For this review, take the finished solid that the model builds, in its own axes (mm). Face numbers are marked on the shaded views. Round coordinates to 2 decimals unless told otherwise and drop trailing zeros. Order: outer loops, then holes, each group sorted by start corner. A loop starts at its lowest first (then second) coordinate and runs counter-clockwise, first axis right, second up. Notation, with made-up numbers: (-22.5, 54.25) -> (17.5, 54.25) arc R27 cw to (17.5, 73.25) -> close; hole circle Ø3 at (55, 78). An arc over 180 degrees is marked (long way). Answer in a Markdown table with one row per item.
```python
from build123d import *

# Parameters (mm, degrees)
SKETCH1_W           = 99
SKETCH1_H           = 51
BOSS_EXTRUDE2_DEPTH = 31
CUT_EXTRUDE1_DEPTH  = 96
SKETCH4_W           = 3
SKETCH4_H           = 31
CUT_EXTRUDE2_DEPTH  = 3
SKETCH6_W           = 2
SKETCH6_H           = 2
BOSS_EXTRUDE3_DEPTH = 96
SKETCH7_W           = 1
SKETCH7_H           = 1
CUT_EXTRUDE3_DEPTH  = 45
FILLET1_R           = 3
SKETCH9_R           = 1
SKETCH9_R_2         = 0.5
CUT_EXTRUDE4_DEPTH  = 10


with BuildPart() as part:
    # Sketch1 → Boss-Extrude2 (new body)
    with BuildSketch(Plane.XY):
        Rectangle(SKETCH1_W, SKETCH1_H)
    extrude(amount=BOSS_EXTRUDE2_DEPTH)

    # Sketch3 → Cut-Extrude1 (cut)
    with BuildSketch(Plane.ZY.offset(49.5)):
        Polygon((3, 0.616456183), (3, -22.5), (28, -22.5), (28, 22.5), (3, 22.5), align=None)
    extrude(amount=-CUT_EXTRUDE1_DEPTH, mode=Mode.SUBTRACT)

    # Sketch4 → Cut-Extrude2 (cut)
    with BuildSketch(Plane.XZ.offset(25.5)):
        with Locations((-48, 15.5)):
            Rectangle(SKETCH4_W, SKETCH4_H)
    extrude(amount=-CUT_EXTRUDE2_DEPTH, mode=Mode.SUBTRACT)

    # Sketch6 → Boss-Extrude3 (add)
    with BuildSketch(Plane.ZY.offset(46.5)):
        with Locations((13.2, -21.5)):
            Rectangle(SKETCH6_W, SKETCH6_H)
        with Locations((17.8, -21.5)):
            Rectangle(SKETCH6_W, SKETCH6_H)
        with Locations((13.2, 21.5)):
            Rectangle(SKETCH6_W, SKETCH6_H)
        with Locations((17.8, 21.5)):
            Rectangle(SKETCH6_W, SKETCH6_H)
    extrude(amount=-BOSS_EXTRUDE3_DEPTH)

    # Sketch7 → Cut-Extrude3 (cut)
    with BuildSketch(Plane.XZ.offset(22.5)):
        with Locations((-48.055142405, 28.5)):
            Rectangle(SKETCH7_W, SKETCH7_H)
        with Locations((-48.055142405, 2.5)):
            Rectangle(SKETCH7_W, SKETCH7_H)
    extrude(amount=-CUT_EXTRUDE3_DEPTH, mode=Mode.SUBTRACT)

    # Fillet1
    fillet1_edges = [part.edges().sort_by_distance(p)[0] for p in [
        (0, 25.5, 31),
        (1.5, -25.5, 31),
        (1.5, -25.5, 0),
        (0, 25.5, 0),
    ]]
    fillet(fillet1_edges, radius=FILLET1_R)

    # Sketch9 → Cut-Extrude4 (cut)
    # profile 1 of 8: a face of its own
    with BuildSketch(Plane(origin=(0, 0, 28), x_dir=(-1, 0, 0), z_dir=(0, 0, -1))):
        with BuildLine():
            ThreePointArc((-43.107346254, 2.807819217), (-44.043005412, 0.051456221), (-43.107346254, -2.704906774))
            ThreePointArc((-43.107346254, -2.704906774), (-42.125865916, -2.834121112), (-41.996651578, -1.852640773))
            ThreePointArc((-41.996651578, -1.852640773), (-42.643005412, 0.051456221), (-41.996651578, 1.955553216))
            ThreePointArc((-41.996651578, 1.955553216), (-42.125865916, 2.937033554), (-43.107346254, 2.807819217))
        make_face()
    # profile 2 of 8: a face of its own
    with BuildSketch(Plane(origin=(0, 0, 28), x_dir=(-1, 0, 0), z_dir=(0, 0, -1))):
        with BuildLine():
            ThreePointArc((-37.730978714, 6.710201232), (-42.153265918, 6.420349215), (-45.485251514, 3.498276272))
            ThreePointArc((-45.485251514, 3.498276272), (-45.229033732, 2.542058489), (-44.272815949, 2.798276272))
            ThreePointArc((-44.272815949, 2.798276272), (-41.617509112, 5.12691787), (-38.093325377, 5.357905075))
            ThreePointArc((-38.093325377, 5.357905075), (-37.236003967, 5.852879822), (-37.730978714, 6.710201232))
        make_face()
    # profile 3 of 8: a face of its own
    with BuildSketch(Plane(origin=(0, 0, 28), x_dir=(-1, 0, 0), z_dir=(0, 0, -1))):
        with BuildLine():
            ThreePointArc((-35.59397575, 2.315366896), (-35.850193532, 1.359149114), (-36.806411315, 1.615366896))
            ThreePointArc((-36.806411315, 1.615366896), (-38.318218652, 2.941186348), (-40.324723797, 3.072699643))
            ThreePointArc((-40.324723797, 3.072699643), (-41.182045207, 3.56767439), (-40.68707046, 4.4249958))
            ThreePointArc((-40.68707046, 4.4249958), (-37.782461847, 4.234617693), (-35.59397575, 2.315366896))
        make_face()
    # profile 4 of 8: a face of its own
    with BuildSketch(Plane(origin=(0, 0, 28), x_dir=(-1, 0, 0), z_dir=(0, 0, -1))):
        with BuildLine():
            ThreePointArc((-34.046091661, -4.145125978), (-32.621543961, 0.051456221), (-34.046091661, 4.24803842))
            ThreePointArc((-34.046091661, 4.24803842), (-35.027572, 4.377252758), (-35.156786338, 3.39577242))
            ThreePointArc((-35.156786338, 3.39577242), (-34.021543961, 0.051456221), (-35.156786338, -3.292859977))
            ThreePointArc((-35.156786338, -3.292859977), (-35.027572, -4.274340315), (-34.046091661, -4.145125978))
        make_face()
    # profile 5 of 8: a face of its own
    with BuildSketch(Plane(origin=(0, 0, 28), x_dir=(-1, 0, 0), z_dir=(0, 0, -1))):
        with BuildLine():
            ThreePointArc((-40.203971578, -4.423668127), (-37.337352845, -3.918205901), (-35.370817206, -1.772108839))
            ThreePointArc((-35.370817206, -1.772108839), (-35.729612558, -0.849468121), (-36.652253276, -1.208263474))
            ThreePointArc((-36.652253276, -1.208263474), (-38.010737122, -2.690788443), (-39.990998837, -3.039962012))
            ThreePointArc((-39.990998837, -3.039962012), (-40.789338265, -3.625328699), (-40.203971578, -4.423668127))
        make_face()
    # profile 6 of 8: a face of its own
    with BuildSketch(Plane(origin=(0, 0, 28), x_dir=(-1, 0, 0), z_dir=(0, 0, -1))):
        with BuildLine():
            ThreePointArc((-46.089765479, -2.021501337), (-45.632657673, -1.143405411), (-44.754561748, -1.600513217))
            ThreePointArc((-44.754561748, -1.600513217), (-42.666206574, -4.448670298), (-39.275554847, -5.436955151))
            ThreePointArc((-39.275554847, -5.436955151), (-38.54568752, -6.105755335), (-39.214487704, -6.835622662))
            ThreePointArc((-39.214487704, -6.835622662), (-43.469213585, -5.59548316), (-46.089765479, -2.021501337))
        make_face()
    # profile 7 of 8: a face of its own
    with BuildSketch(Plane(origin=(0, 0, 28), x_dir=(-1, 0, 0), z_dir=(0, 0, -1))):
        with Locations((-39.515184062, 0.051456221)):
            Circle(SKETCH9_R)
        with Locations((-39.515184062, 0.051456221)):
            Circle(SKETCH9_R_2, mode=Mode.SUBTRACT)
    # profile 8 of 8: a face of its own
    with BuildSketch(Plane(origin=(0, 0, 28), x_dir=(-1, 0, 0), z_dir=(0, 0, -1))):
        with Locations((-39.515184062, 0.051456221)):
            Circle(SKETCH9_R_2)
    extrude(amount=-CUT_EXTRUDE4_DEPTH, mode=Mode.SUBTRACT)


solid = part.part
```
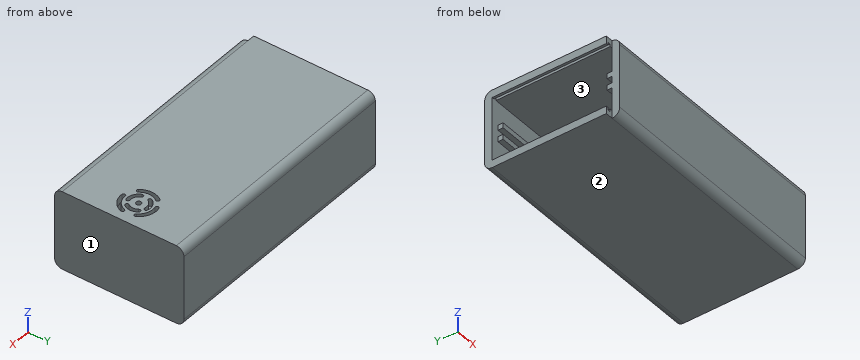
Q1. To check wall thickness, follow probe 1 along Y at (x, z) = (-32.5, 22); probe 2 along Z at (x, y) = (-42.5, -22); probe 3 along Z at (x, y) = (28, 8). State the ranges of each line that lie inside material, in increasing order.
Answer key:
| item | result |
|---|---|
| probe 1 | y = -25.5 to -22.5, 22.5 to 25.5 |
| probe 2 | z = 0 to 3, 12.2 to 14.2, 16.8 to 18.8, 28 to 31 |
| probe 3 | z = 0 to 3, 28 to 31 |
Q2. Take a section at A-A, the plane x = -12.5. Write out the cut boundary in (y, z).
Answer key:
| item | result |
|---|---|
| outline | (-25.5, 3) arc R3 ccw to (-22.5, 0) -> (22.5, 0) arc R3 ccw to (25.5, 3) -> (25.5, 28) arc R3 ccw to (22.5, 31) -> (-22.5, 31) arc R3 ccw to (-25.5, 28) -> close; hole (-22.5, 3) -> (22.5, 3) -> (22.5, 12.2) -> (20.5, 12.2) -> (20.5, 14.2) -> (22.5, 14.2) -> (22.5, 16.8) -> (20.5, 16.8) -> (20.5, 18.8) -> (22.5, 18.8) -> (22.5, 28) -> (-22.5, 28) -> (-22.5, 18.8) -> (-20.5, 18.8) -> (-20.5, 16.8) -> (-22.5, 16.8) -> (-22.5, 14.2) -> (-20.5, 14.2) -> (-20.5, 12.2) -> (-22.5, 12.2) -> close |
Q3. Clearance check with flat-ended pins moving along their axes: pin 1 Ø0.9 at (x, z) = (-47.5, 1) entering from -Y; pin 2 Ø4 at (y, z) = (18.5, 21) entering from -X; pin 3 Ø2 at (y, z) = (21, 17.5) entering from -X. State where each tip first meets the part, or that it passes through.
Answer key:
| item | result |
|---|---|
| pin 1 | stops at y = -22.5 |
| pin 2 | stops at x = 46.5 |
| pin 3 | stops at x = -46.5 |
Q4. The part is to be moulded in two halves that separate along Z. For the marked faces 1, 2 and 3, say which applies: +Z half, -Z half, draft (parallel to the pull), parting line (faces both ways), or undercut.
Answer key:
| item | result |
|---|---|
| face 1 | draft |
| face 2 | -Z half |
| face 3 | undercut |
Q5. Take a section at B-B, the plane z = 5. Write out the cut boundary in (x, y).
Answer key:
| item | result |
|---|---|
| outline | (-49.5, 22.5) -> (46.5, 22.5) -> (46.5, -22.5) -> (-46.5, -22.5) -> (-46.5, -25.5) -> (49.5, -25.5) -> (49.5, 25.5) -> (-49.5, 25.5) -> close |
Q6. Take a section at C-C, the plane y = 8. Write out the cut boundary in (x, z).
Answer key:
| item | result |
|---|---|
| outline | (-49.5, 0) -> (49.5, 0) -> (49.5, 31) -> (-49.5, 31) -> (-49.5, 28) -> (-48.56, 28) -> (-48.56, 29) -> (-47.56, 29) -> (-47.56, 28) -> (46.5, 28) -> (46.5, 3) -> (-47.56, 3) -> (-47.56, 2) -> (-48.56, 2) -> (-48.56, 3) -> (-49.5, 3) -> close |
